Build history of the part. All positions in model axes, mm. A direction names the side the tool comes from. Give positions to 0.01 mm unless a question says otherwise; leave off trailing zeros. Loops run counter-clockwise (first coordinate to the right, second up) from the corner with the lowest first, then second, coordinate; pieces in that order, holes last.
1) Band-saw the part on B-B on y = 0.25. State how many separate pieces and enclosed holes the cut face has, then the cut area to 3 significant figures.
2) Flat gauge pins, fed straight in: P1, Ø4, axis at x = 18, y = -4.5, coming from the +Z side (3 decimals); P2, Ø5, axis at x = 16.5, z = -2, coming from the -Y side; P3, Ø3.5, axis at x = 9.525, y = 0, coming from the +Z side; P4, Ø4, axis at x = 18.26, y = 0, coming from the -Z side. Where does each tip first touch, or does it go through?
3) Two-plate mould, pull along X, no slides. Class faces 4 (the flat face through (16, -2, -3.175)), 5 (the conical face through (5.475, 0.197, -5.434)), 6 (the conical face through (22.054, 4.303, 0.053)): +X half, -X half, draft (parallel to the pull), parting line (faces both ways), or undercut.
4) Wall check: line 1 (X direction, y = 0, z = 2.1) (3 decimals); line 2 (Z direction, x = 6.5, y = 0); line 3 (X direction, y = 2.5, z = 3.75). Give the ranges that are in metal, low to high.
5) 3-axis set-ups, long thin cutter, end or side, ignore diameter. For faces 1 (the cylindrical face through (1.725, -0.885, 3.986)), 2 (the cylindrical face through (17.629, 4.762, 0.049)), 3 (the cylindrical face through (17.629, -4.762, -0.049)): which of +Z, -Z, +X, -X, +Y, -Y reach the whole face in a straight line?
6) Band-saw the part on A-A on x = 17.5. List the corners of the cut face in (y, z) (1 decimal), then the cut area to 3 significant figures.
```python
from build123d import *

# Parameters (mm, degrees)
SKETCH3_W               = 22.2504
SKETCH3_H               = 44.5008
SKETCH3_W_2             = 6.35
SKETCH3_H_2             = 22.2504
CUT_EXTRUDE1_DEPTH      = 8.6741
SKETCH4_W               = 5.5626
SKETCH4_H               = 11.1252
CUT_EXTRUDE2_DEPTH      = 8.2042
HOLE1_D                 = 3.96748
HOLE1_DEPTH             = 13.5509
HOLE1_TIP               = 1.145312823
HOLE2_D                 = 3.96748
HOLE2_DEPTH             = 4.5339
HOLE2_CSINK_D           = 4.826
HOLE2_CSINK_ANGLE       = 90
SKETCH10_R              = 2.40665
CUT_EXTRUDE3_DEPTH      = 4.7625
CUT_EXTRUDE3_DEPTH_BACK = 4.7625


with BuildPart() as part:
    # Sketch1 → Revolve1 (revolve)
    with BuildSketch(Plane.XY):
        Polygon((0, 0), (0, 3.57505), (0.508, 4.08305), (2.9083, 4.08305), (3.4671, 3.52425), (4.0259, 3.52425), (4.0259, 4.3053), (4.2799, 4.5593), (5.3467, 4.5593), (5.3467, 5.3086), (5.6007, 5.5626), (13.2969, 5.5626), (13.5509, 5.3086), (13.5509, 0), align=None)
    revolve(axis=Axis((13.5509, 0, 0), (-1, 0, 0)))

    # Sketch2 → Revolve2 (revolve)
    with BuildSketch(Plane.XY):
        Polygon((13.5509, 0), (13.5509, 4.7625), (21.59508, 4.7625), (22.225, 4.13258), (22.225, 0), align=None)
    revolve(axis=Axis((22.225, 0, 0), (-1, 0, 0)))

    # Sketch3 → Cut-Extrude1 (cut)
    with BuildSketch(Plane(origin=(22.225, 0, 0), x_dir=(0, 0, -1), z_dir=(1, 0, 0))):
        Rectangle(SKETCH3_W, SKETCH3_H)
        Rectangle(SKETCH3_W_2, SKETCH3_H_2, mode=Mode.SUBTRACT)
    extrude(amount=-CUT_EXTRUDE1_DEPTH, mode=Mode.SUBTRACT)

    # Sketch4 → Cut-Extrude2 (cut)
    with BuildSketch(Plane(origin=(13.5509, 0, 0), x_dir=(0, 0, -1), z_dir=(1, 0, 0))):
        with Locations((-7.3152, 0)):
            Rectangle(SKETCH4_W, SKETCH4_H)
    extrude(amount=-CUT_EXTRUDE2_DEPTH, mode=Mode.SUBTRACT)

    # Hole1
    with Locations(Plane.ZY):
        with Locations((0, 0)):
            Hole(HOLE1_D / 2, depth=HOLE1_DEPTH)
            with Locations((0, 0, -(HOLE1_DEPTH + HOLE1_TIP / 2))):  # 120° drill point
                Cone(0, HOLE1_D / 2, HOLE1_TIP, mode=Mode.SUBTRACT)

    # Hole2
    with Locations(Plane.XY.offset(4.5339)):
        with Locations((9.525, 0)):
            CounterSinkHole(HOLE2_D / 2, HOLE2_CSINK_D / 2, depth=HOLE2_DEPTH, counter_sink_angle=HOLE2_CSINK_ANGLE)

    # Sketch9 → Revolve3 (revolve)
    with BuildSketch(Plane.XY):
        with BuildLine():
            Line((3.306480735, 4.475131804), (3.912128708, 3.869483831))
            ThreePointArc((3.912128708, 3.869483831), (3.949326147, 3.779681269), (3.912128708, 3.689878708))
            Line((3.912128708, 3.689878708), (3.7465, 3.52425))
            Line((3.7465, 3.52425), (3.4671, 3.52425))
            Line((3.4671, 3.52425), (3.4671, 3.27025))
            Line((3.4671, 3.27025), (4.0259, 3.27025))
            Line((4.0259, 3.27025), (4.0259, 4.043080735))
            Line((4.0259, 4.043080735), (3.509680735, 4.5593))
            Line((3.509680735, 4.5593), (3.306480735, 4.5593))
            Line((3.306480735, 4.5593), (3.306480735, 4.475131804))
        make_face()
    revolve(axis=Axis((4.0259, 0, 0), (-1, 0, 0)))

    # Sketch10 → Cut-Extrude3 (cut, two sides)
    with BuildSketch(Plane.XY) as cut_extrude3_sk:
        with Locations((18.2626, 0)):
            Circle(SKETCH10_R)
    extrude(amount=CUT_EXTRUDE3_DEPTH, mode=Mode.SUBTRACT)
    extrude(cut_extrude3_sk.sketch, amount=-CUT_EXTRUDE3_DEPTH_BACK, mode=Mode.SUBTRACT)


solid = part.part
```
Findings below:
1. separate pieces: 3
1. enclosed holes: 0
1. area: 85.7 mm2
2. P1: stops at z = 3.175
2. P2: stops at y = -4.76
2. P3: stops at z = -0.93
2. P4: passes through
3. face 4: draft
3. face 5: -X half
3. face 6: +X half
4. line 1: x = 0 to 7.541, 11.509 to 15.856, 20.669 to 22.225
4. line 2: z = -5.56 to -1.98, 1.98 to 4.53
4. line 3: x = 3.31 to 3.56, 4.23 to 13.55
5. face 1: -X
5. face 2: +X, +Y
5. face 3: +X, -Y
6. outline: (-3.5, -3.2) - (-2.3, -3.2) - (-2.3, 3.2) - (-3.5, 3.2) arc R4.8 ccw to start; (2.3, -3.2) - (3.5, -3.2) arc R4.8 ccw to (3.5, 3.2) - (2.3, 3.2) - close
6. area: 26.7 mm2
